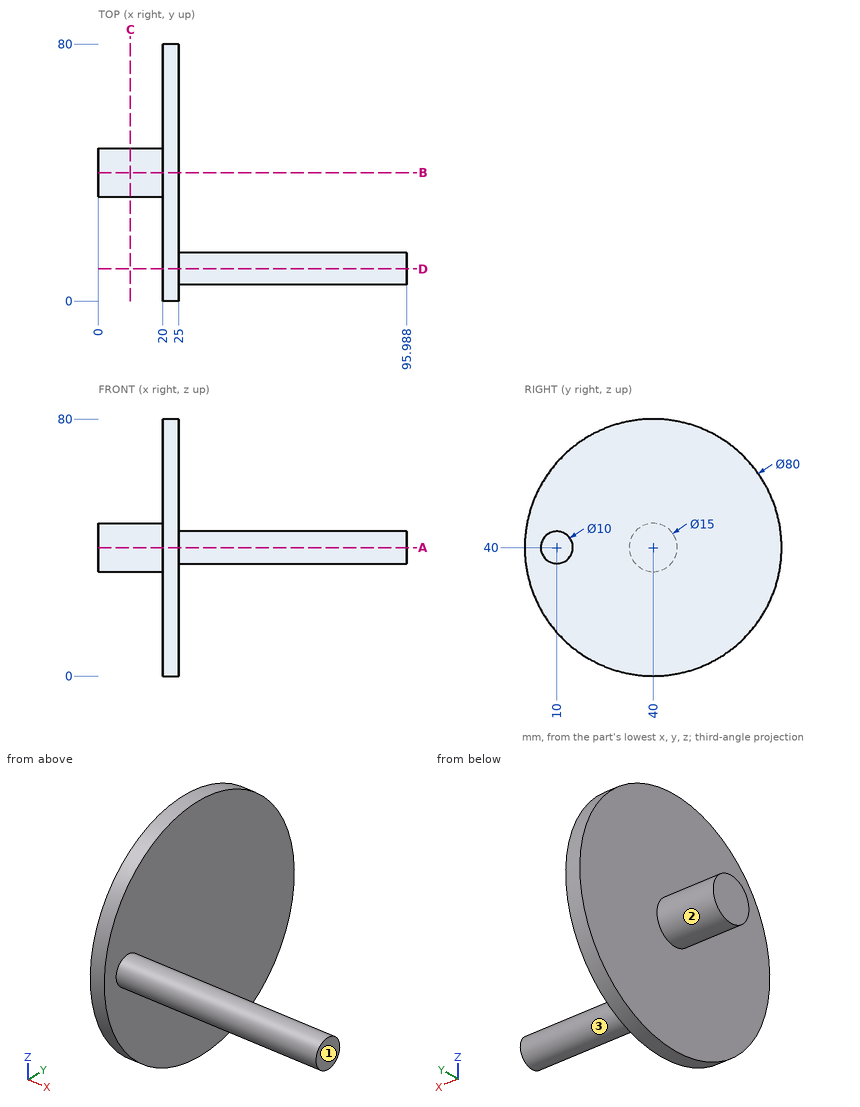
Source: three-view drawing plus pictorial views. Frame: mm from the lowest corner of the part. A direction names the side the tool comes from. Round coordinates to 2 decimals unless told otherwise and drop trailing zeros. Write each loop counter-clockwise with the first axis right and the second up, starting at its lowest first coordinate (ties: lowest second). Pieces come first, ordered by that corner, then holes. Notation, with made-up numbers: M 20,-12 L 39,-12 A31 ccw 39,15 Z; hole C -16.75,-1.5 d11. An arc over 180 degrees is marked long. Use CSV: the item, a comma, the result in double quotes. Start each with the question number.
Q1. Cut plane A-A on z = 40. Output: boundary loops of the cut face in (x, y).
Q2. Cut plane B-B on y = 40. Output: boundary loops of the cut face in (x, z).
Q3. Cut plane D-D on y = 10. Output: boundary loops of the cut face in (x, z), plus the area to 3 significant figures.
Q4. Cut plane C-C on x = 10. Output: boundary loops of the cut face in (y, z).
Q5. Access query for the marked faces 1, 2 and 3. Directions: +Z, -Z, +X, -X, +Y, -Y. A direction counts if a zero-diameter tool reaches every point of the face in a straight line with its end or side. Return the directions, or none.
Q6. Line query: line 1 (X direction, y = 75, z = 34); line 2 (X direction, y = 12, z = 37); line 3 (Y direction, x = 13, z = 46). Output: solid intervals per line, ascending. Write a range as from..to.
Q7. First-contact query: P1, Ø3, axis at x = 25, z = 62.5, coming from the -Y side; P2, Ø3, axis at x = 43.5, z = 44, coming from the -Y side; P3, Ø12, axis at x = 17.5, y = 20.5, coming from the -Z side; P4, Ø10, axis at x = 31.5, z = 67, coming from the -Y side. Flat tips, straight axial feed; report the tip coordinate or a pass-through.
Results found:
1,outline,"M 0,32.5 L 20,32.5 L 20,0 L 25,0 L 25,5 L 95.99,5 L 95.99,15 L 25,15 L 25,80 L 20,80 L 20,47.5 L 0,47.5 Z"
2,outline,"M 0,32.5 L 20,32.5 L 20,0 L 25,0 L 25,80 L 20,80 L 20,47.5 L 0,47.5 Z"
3,outline,"M 20,13.54 L 25,13.54 L 25,35 L 95.99,35 L 95.99,45 L 25,45 L 25,66.46 L 20,66.46 Z"
3,area,"974 mm^2"
4,outline,"C 40,40 d15"
5,face 1,"+Z, -Z, +X, +Y, -Y"
5,face 2,"-X"
5,face 3,"+X"
6,line 1,"20..25"
6,line 2,"20..95.99"
6,line 3,"35.5..44.5"
7,P1,"y = 5.96"
7,P2,"y = 5.67"
7,P3,"z = 2.55"
7,P4,"through"
